For this review, use the dimensioned drawing (mm, ordinates from the lowest corner) and the shaded views. A direction names the side the tool comes from. Round coordinates to 2 decimals unless told otherwise and drop trailing zeros. Write each loop counter-clockwise with the first axis right and the second up, starting at its lowest first coordinate (ties: lowest second). Pieces come first, ordered by that corner, then holes. Notation, with made-up numbers: (46.25, 37) - (69.25, 37) arc R22 ccw to (69.25, 57) - close; hole circle Ø9 at (-26, 55). An arc over 180 degrees is marked (long way). Return JSON: item names as keys, results as strings.
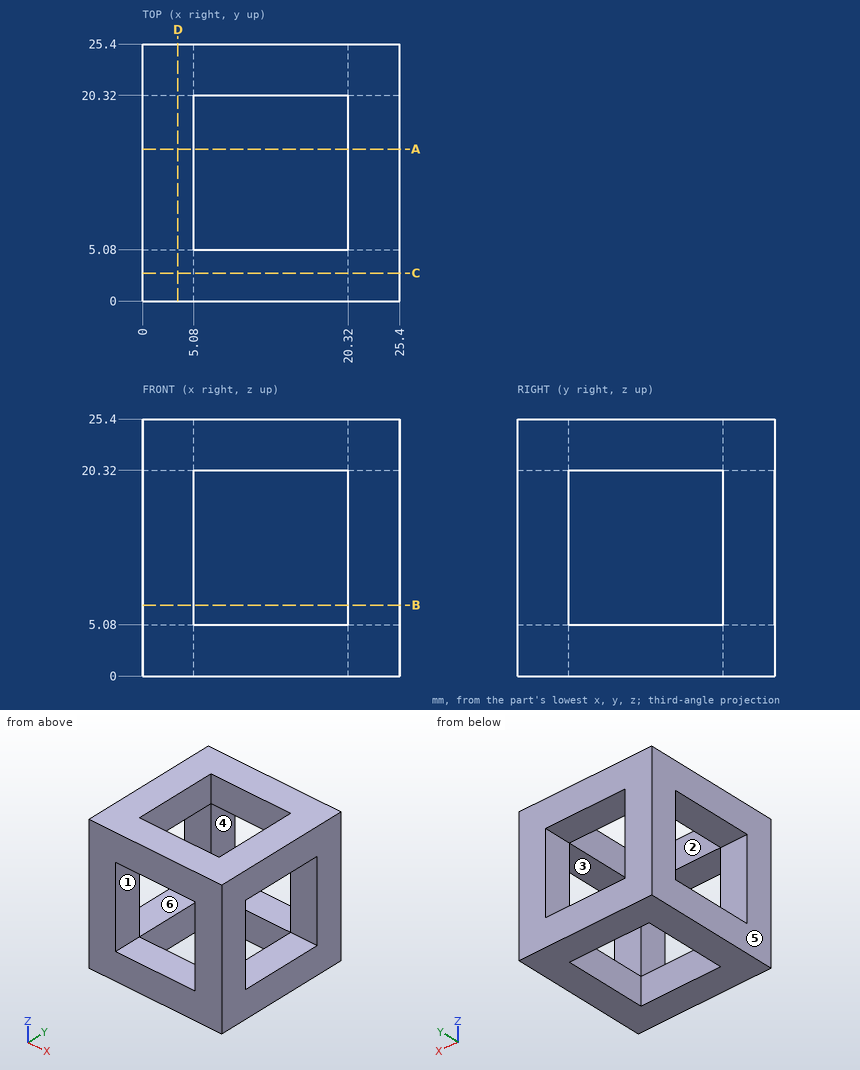
(1) Wall thickness on line 1 (X direction, y = 20, z = 1.5): over which ranges is the line inside the solid? List them lowest first.
Filled in:
{"line 1": "x = 0 to 5.08, 20.32 to 25.4"}
(2) Clearance check with a flat-ended pin moving along its axis: pin 1 Ø8 at (x, y) = (13.5, 11.5) entering from -Z. State where the tip first meets the part, or that it passes through.
Filled in:
{"pin 1": "passes through"}
(3) For the marked faces 1, 2 and 3, list the 3-axis set-ups (+Z, -Z, +X, -X, +Y, -Y) from which the entire face can be reached by the end or side of a thin tool; tool diameter is ignored.
Filled in:
{"face 1": "+Y, -Y", "face 2": "+Z, -Z", "face 3": "+X, -X"}
(4) Mouldability with a two-part tool opening along X and no side actions: class the marked faces 4, 5 and 6 as released by +X, released by -X, zero draft, split by the parting line, or undercut.
Filled in:
{"face 4": "undercut", "face 5": "released by -X", "face 6": "zero draft"}
(5) Add section A-A (y = 15). Write out the cut boundary in (x, z), plus the area to 3 significant figures.
Filled in:
{"outline": "(0, 0) - (5.08, 0) - (5.08, 5.08) - (0, 5.08) - close; (0, 20.32) - (5.08, 20.32) - (5.08, 25.4) - (0, 25.4) - close; (20.32, 0) - (25.4, 0) - (25.4, 5.08) - (20.32, 5.08) - close; (20.32, 20.32) - (25.4, 20.32) - (25.4, 25.4) - (20.32, 25.4) - close", "area": "103 mm2"}
(6) Add section C-C (y = 2.75). Write out the cut boundary in (x, z).
Filled in:
{"outline": "(0, 0) - (25.4, 0) - (25.4, 25.4) - (0, 25.4) - close; hole (5.08, 5.08) - (20.32, 5.08) - (20.32, 20.32) - (5.08, 20.32) - close"}
